Study the drawing (mm; zero at the part's minimum x, y, z) and answer. Round coordinates to 2 decimals unless told otherwise and drop trailing zeros. Write each loop counter-clockwise with the first axis right and the second up, starting at its lowest first coordinate (ties: lowest second). Pieces come first, ordered by that corner, then holes.
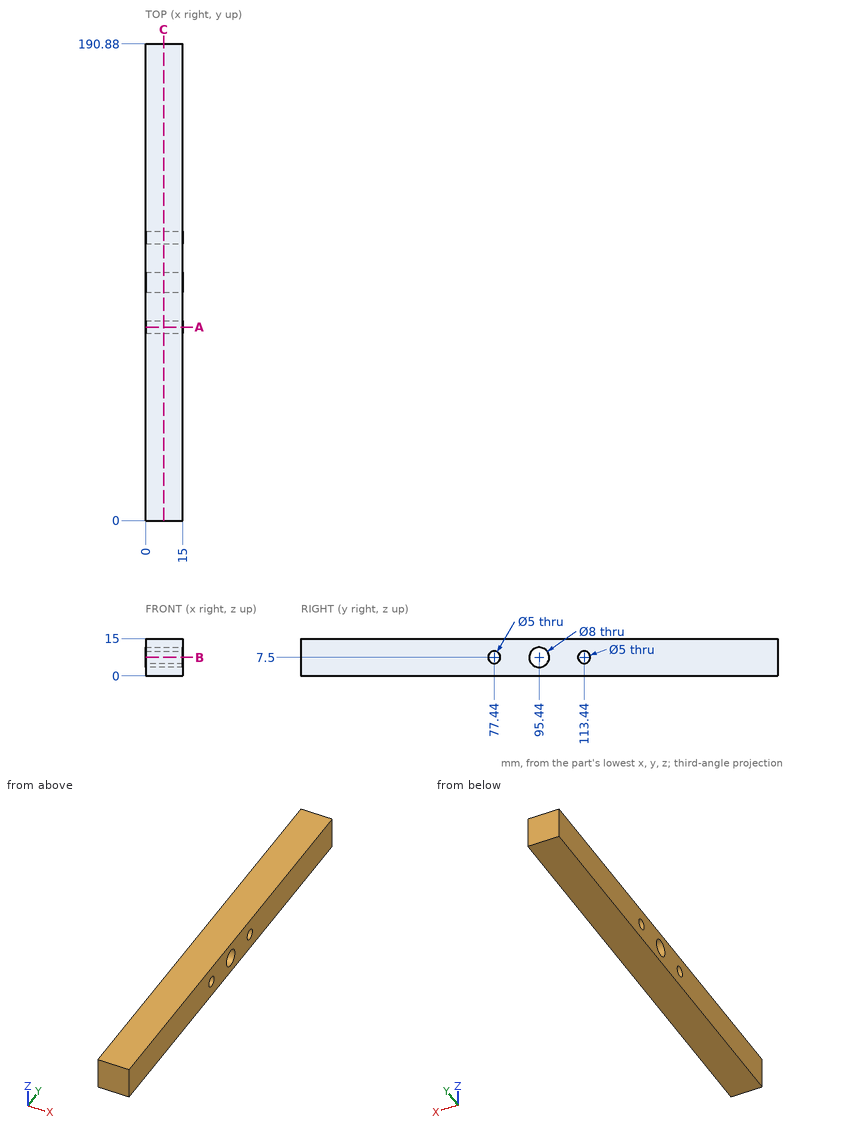
1. Section B-B on z = 7.5 is taken. Determine the outline of the cut face in (x, y), plus the area to 3 significant figures.
Geometry says:
outline: (0, 0) - (15, 0) - (15, 74.94) - (0, 74.94) - close; (0, 79.94) - (15, 79.94) - (15, 91.44) - (0, 91.44) - close; (0, 99.44) - (15, 99.44) - (15, 110.94) - (0, 110.94) - close; (0, 115.94) - (15, 115.94) - (15, 190.88) - (0, 190.88) - close
area: 2,590 mm2
2. Straight lines are drawn through the part: line 1 along Y through (x, z) = (4.25, 7.5); line 2 along Y through (x, z) = (1.25, 9.75); line 3 along Y through (x, z) = (8, 4). For each, find the intervals that lie inside material, in ascending order.
Geometry says:
line 1: y = 0 to 74.94, 79.94 to 91.44, 99.44 to 110.94, 115.94 to 190.88
line 2: y = 0 to 76.35, 78.53 to 92.13, 98.75 to 112.35, 114.53 to 190.88
line 3: y = 0 to 93.5, 97.38 to 190.88
3. Given pin 1 (3 mm diameter, centred on y = 77.44, z = 7.5, fed in from +X); pin 2 (4 mm diameter, centred on x = 5.5, y = 120.5, fed in from -Z), each flat-ended and moving along its own axis, determine where each tip first touches the part or whether it passes through.
Geometry says:
pin 1: passes through
pin 2: stops at z = 0
4. Section A-A on y = 77.44 is taken. Determine the outline of the cut face in (x, z).
Geometry says:
outline: (0, 0) - (15, 0) - (15, 5) - (0, 5) - close; (0, 10) - (15, 10) - (15, 15) - (0, 15) - close
5. Section C-C on x = 7.25 is taken. Determine the outline of the cut face in (y, z), plus the area to 3 significant figures.
Geometry says:
outline: (0, 0) - (190.88, 0) - (190.88, 15) - (0, 15) - close; hole circle Ø5 at (77.44, 7.5); hole circle Ø8 at (95.44, 7.5); hole circle Ø5 at (113.44, 7.5)
area: 2,770 mm2
